Geometry check sheet. Reference: the model listing, model coordinates, mm. Face numbers are marked on the shaded views. A direction names the side the tool comes from. Round coordinates to 2 decimals unless told otherwise and drop trailing zeros. Loops run counter-clockwise (first coordinate to the right, second up) from the corner with the lowest first, then second, coordinate; pieces in that order, holes last. Notation, with made-up numbers: M 64,18 L 70,18 A21 cw 70,30 Z; hole C 4.5,-25 d3. An arc over 180 degrees is marked long. Use one line per item in the form item = value. Start each with the question number.
1. Cross-section at A-A (y = 5). Record the boundary of the cut face in (x, z).
2. Cross-section at B-B (y = 7). Record the boundary of the cut face in (x, z), then the cut area to 3 significant figures.
3. Material ranges on line 1 (X direction, y = 2.5, z = -2.5); line 2 (Y direction, x = 6, z = -6.5); line 3 (Y direction, x = 2.7, z = -5), recorded low to high.
4. Cross-section at D-D (z = -7). Record the boundary of the cut face in (x, y), then the cut area to 3 significant figures.
5. Cross-section at C-C (x = 6). Record the boundary of the cut face in (y, z).
6. Go/stop test with flat-tipped pins: pin 1 (1.8 mm diameter, centred on x = 6, y = 5, fed in from +Z); pin 2 (1.7 mm diameter, centred on x = 13.5, z = -4, fed in from +Y); pin 3 (0.7 mm diameter, centred on x = 12, y = 9, fed in from +Z). Record where each tip stops, or that it passes through.
7. Set-up check for the marked faces 1, 2 and 3: record each of +Z, -Z, +X, -X, +Y, -Y from which the full face is reachable in a straight line by a thin tool's end or side.
8. Draft check along X on the marked faces 4, 5, 6 and 7. Enter one of: pulls with the +X half, pulls with the -X half, needs draft (parallel to the pull), parting line crosses it, or undercut.
```python
from build123d import *

# Parameters (mm, degrees)
SKETCH1_W           = 74.5
SKETCH1_H           = 10
BOSS_EXTRUDE1_DEPTH = 10
SKETCH2_R           = 1.25
CUT_EXTRUDE1_DEPTH  = 10
SKETCH4_R           = 1.25
CUT_EXTRUDE3_DEPTH  = 5
CUT_EXTRUDE4_START  = -12
SKETCH5_R           = 1.25
CUT_EXTRUDE4_DEPTH  = 12
CUT_EXTRUDE5_DEPTH  = 2.2
CUT_EXTRUDE6_DEPTH  = 2.2
SKETCH11_W          = 2.3
SKETCH11_H          = 5.6
CUT_EXTRUDE9_DEPTH  = 7.3
SKETCH12_W          = 92.79599186
SKETCH12_H          = 35.188487641
CUT_EXTRUDE10_DEPTH = 14
SKETCH13_W          = 8.109024166
SKETCH13_H          = 12.314563919
CUT_EXTRUDE11_DEPTH = 12
FILLET2_R           = 2
FILLET3_R           = 2


with BuildPart() as part:
    # Sketch1 → Boss-Extrude1 (new body)
    with BuildSketch(Plane(origin=(0, 0, 0), x_dir=(1, 0, 0), z_dir=(0, 1, 0))):
        with Locations((37.25, 5)):
            Rectangle(SKETCH1_W, SKETCH1_H)
    extrude(amount=BOSS_EXTRUDE1_DEPTH)

    # Sketch2 → Cut-Extrude1 (cut)
    with BuildSketch(Plane(origin=(0, 10, 0), x_dir=(1, 0, 0), z_dir=(0, 1, 0))):
        with Locations(Location((12, 5, 0), (0, 0, 270))):
            Circle(SKETCH2_R)
        with Locations(Location((62.5, 5, 0), (0, 0, 270))):
            Circle(SKETCH2_R)
    extrude(amount=-CUT_EXTRUDE1_DEPTH, mode=Mode.SUBTRACT)

    # Sketch4 → Cut-Extrude3 (cut)
    with BuildSketch(Plane(origin=(74.5, 0, 0), x_dir=(0, 0, -1), z_dir=(1, 0, 0))):
        with Locations((5, 5)):
            Circle(SKETCH4_R)
    extrude(amount=-CUT_EXTRUDE3_DEPTH, mode=Mode.SUBTRACT)

    # Sketch5 → Cut-Extrude4 (cut)
    with BuildSketch(Plane.ZY.offset(CUT_EXTRUDE4_START)):
        with Locations(Location((-5, 5, 0), (0, 0, 180))):
            Circle(SKETCH5_R)
    extrude(amount=CUT_EXTRUDE4_DEPTH, mode=Mode.SUBTRACT)

    # Sketch6 → Cut-Extrude5 (cut)
    with BuildSketch(Plane(origin=(0, 10, 0), x_dir=(1, 0, 0), z_dir=(0, 1, 0))):
        Polygon((13.616580754, 2.2), (15.233161507, 5), (13.616580754, 7.8), (10.383419246, 7.8), (8.766838493, 5), (10.383419246, 2.2), align=None)
    extrude(amount=-CUT_EXTRUDE5_DEPTH, mode=Mode.SUBTRACT)

    # Sketch7 → Cut-Extrude6 (cut)
    with BuildSketch(Plane(origin=(0, 10, 0), x_dir=(1, 0, 0), z_dir=(0, 1, 0))):
        Polygon((60.883419246, 7.8), (59.266838493, 5), (60.883419246, 2.2), (64.116580754, 2.2), (65.733161507, 5), (64.116580754, 7.8), align=None)
    extrude(amount=-CUT_EXTRUDE6_DEPTH, mode=Mode.SUBTRACT)

    # Sketch11 → Cut-Extrude9 (cut)
    with BuildSketch(Plane.XY):
        with Locations((6.15, 5)):
            Rectangle(SKETCH11_W, SKETCH11_H)
        with Locations((68.35, 5)):
            Rectangle(SKETCH11_W, SKETCH11_H)
    extrude(amount=-CUT_EXTRUDE9_DEPTH, mode=Mode.SUBTRACT)

    # Sketch12 → Cut-Extrude10 (cut)
    with BuildSketch(Plane.XY):
        with Locations((72.539564665, 12.110455679)):
            Rectangle(SKETCH12_W, SKETCH12_H)
    extrude(amount=-CUT_EXTRUDE10_DEPTH, mode=Mode.SUBTRACT)

    # Sketch13 → Cut-Extrude11 (cut)
    with BuildSketch(Plane(origin=(0, 10, 0), x_dir=(1, 0, 0), z_dir=(0, 1, 0))):
        with Locations((22.887582964, 5.058087566)):
            Rectangle(SKETCH13_W, SKETCH13_H)
    extrude(amount=-CUT_EXTRUDE11_DEPTH, mode=Mode.SUBTRACT)

    # Fillet2
    fillet2_edges = [part.edges().sort_by_distance(p)[0] for p in [
        (18.833070881, 5, 0),
    ]]
    fillet(fillet2_edges, radius=FILLET2_R)

    # Fillet3
    fillet3_edges = [part.edges().sort_by_distance(p)[0] for p in [
        (18.833070881, 10, -6),
        (18.247284443, 10, -0.585786438),
        (8.416535441, 10, 0),
    ]]
    fillet(fillet3_edges, radius=FILLET3_R)


solid = part.part
```
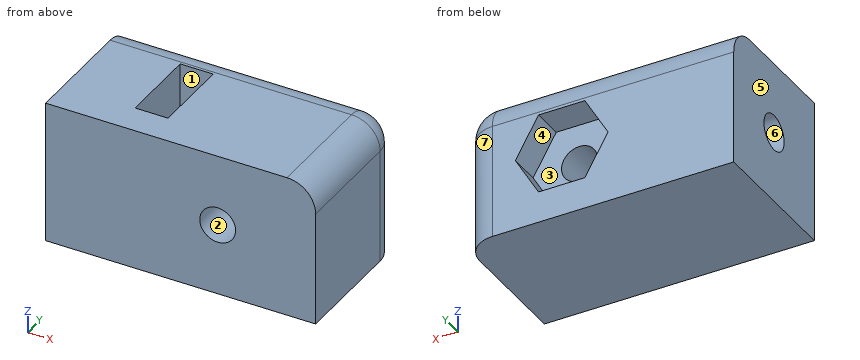
Reported:
q1.outline = M 0,-10 L 18.83,-10 L 18.83,-2 A2 ccw 16.83,0 L 7.3,0 L 7.3,-3.75 L 12,-3.75 A1.25 cw 12,-6.25 L 7.3,-6.25 L 7.3,-7.3 L 5,-7.3 L 5,-6.25 L 0,-6.25 Z; M 0,-3.75 L 5,-3.75 L 5,0 L 0,0 Z
q2.outline = M 0,-10 L 18.83,-10 L 18.83,-2 A2 ccw 16.83,0 L 7.3,0 L 7.3,-7.3 L 5,-7.3 L 5,0 L 0,0 Z; hole C 12,-5 d2.5
q2.area = 166 mm²
q3.line_1 = 0 to 5, 7.3 to 18.83
q3.line_2 = 0 to 2.2, 7.8 to 10
q3.line_3 = 0 to 3.75, 6.25 to 10
q4.outline = M 0,0 L 18.83,0 L 18.83,8 A2 ccw 16.83,10 L 14.08,10 L 14.08,7.8 L 9.92,7.8 L 9.92,10 L 0,10 Z; hole M 5,2.2 L 7.3,2.2 L 7.3,7.8 L 5,7.8 Z
q4.area = 165 mm²
q5.outline = M 0,-10 L 10,-10 L 10,-2 A2 ccw 8,0 L 7.8,0 L 7.8,-7.3 L 2.2,-7.3 L 2.2,0 L 0,0 Z
q6.pin_1 = -7.3
q6.pin_2 = 7.8
q6.pin_3 = -0.11
q7.face_1 = +Z
q7.face_2 = +Y, -Y
q7.face_3 = +Y
q8.face_4 = undercut
q8.face_5 = pulls with the -X half
q8.face_6 = needs draft
q8.face_7 = pulls with the +X half
